Can you work these out from the drawing? Everything is in mm from the part's minimum corner. Round coordinates to 2 decimals unless told otherwise and drop trailing zeros. Order: outer loops, then holes, each group sorted by start corner. A loop starts at its lowest first (then second) coordinate and runs counter-clockwise, first axis right, second up. Notation, with made-up numbers: (-24.75, 70) - (-13.75, 70) arc R19 cw to (-13.75, 98) - close; hole circle Ø5 at (-16, -31). An arc over 180 degrees is marked (long way). Write item = value, one per line.
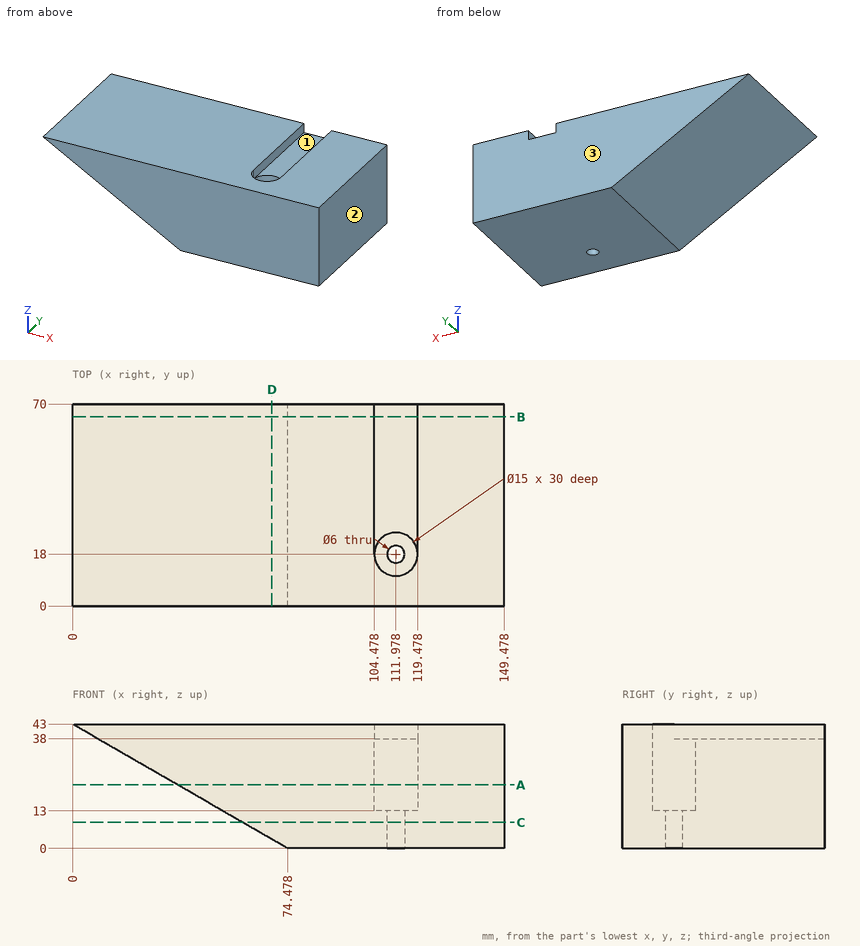
(1) Will these pins go through, and if not, where does the flat tip stop? P1, Ø6, axis at x = 18, z = 26, coming from the -Y side; P2, Ø13.5, axis at x = 111.98, y = 18, coming from the +Z side; P3, Ø12, axis at y = 22.5, z = 19.5, coming from the -X side; P4, Ø1.5, axis at y = 35.5, z = 40.5, coming from the -X side.
Computed:
P1 = through
P2 = 13
P3 = 30.31
P4 = 3.03
(2) If we section it at D-D (x = 69): Write out the boundary of the cut face in (y, z).
Computed:
outline = (0, 3.16) - (70, 3.16) - (70, 43) - (0, 43) - close
(3) If we section it at A-A (z = 22): Write out the boundary of the cut face in (x, y).
Computed:
outline = (36.37, 0) - (149.48, 0) - (149.48, 70) - (36.37, 70) - close; hole circle Ø15 at (111.98, 18)
(4) If we section it at C-C (z = 9): Write out the boundary of the cut face in (x, y).
Computed:
outline = (58.89, 0) - (149.48, 0) - (149.48, 70) - (58.89, 70) - close; hole circle Ø6 at (111.98, 18)
(5) If we section it at B-B (y = 65.5): Write out the boundary of the cut face in (x, z).
Computed:
outline = (0, 43) - (74.48, 0) - (149.48, 0) - (149.48, 43) - (119.48, 43) - (119.48, 38) - (104.48, 38) - (104.48, 43) - close
(6) Thinking about a two-plate mould opening in X: for the marked faces 1, 2 and 3, which applies, +X half, -X half, draft (parallel to the pull), parting line (faces both ways), or undercut?
Computed:
face_1 = undercut
face_2 = +X half
face_3 = draft
(7) If I drill on line 1 (Y direction, x = 112.5, z = 22); line 2 (Z direction, x = 118.5, y = 62); line 3 (X direction, y = 18, z = 20), over which ranges is the centre line in solid material (lowest first)? Write a range as from..to.
Computed:
line_1 = 0..10.52, 25.48..70
line_2 = 0..38
line_3 = 39.84..104.48, 119.48..149.48
